```python
from build123d import *

# Parameters (mm, degrees)
SKETCH1_W           = 72.75
SKETCH1_H           = 35.5
BOSS_EXTRUDE1_DEPTH = 2
SKETCH7_W           = 10.759451316
SKETCH7_H           = 30
BOSS_EXTRUDE4_DEPTH = 4
SKETCH10_W          = 10.759451316
SKETCH10_H          = 10
BOSS_EXTRUDE5_DEPTH = 43.2
FILLET2_R           = 5
SKETCH12_W          = 72.75
SKETCH12_H          = 35.5
BOSS_EXTRUDE6_DEPTH = 2
FILLET4_R           = 2
SKETCH16_W          = 27.8
SKETCH16_H          = 6.7
BOSS_EXTRUDE8_DEPTH = 8
SKETCH19_R          = 1.45
CUT_EXTRUDE2_DEPTH  = 4
SKETCH20_R          = 0.45
CUT_EXTRUDE3_DEPTH  = 102.358708347
SKETCH21_R          = 3.1
CUT_EXTRUDE4_DEPTH  = 5


with BuildPart() as part:
    # Sketch1 → Boss-Extrude1 (new body)
    with BuildSketch(Plane(origin=(0, 0, 0), x_dir=(1, 0, 0), z_dir=(0, 1, 0))):
        with Locations((30.829669563, 14.626919984)):
            Rectangle(SKETCH1_W, SKETCH1_H)
    extrude(amount=BOSS_EXTRUDE1_DEPTH)

    # Sketch7 → Boss-Extrude4 (add)
    with BuildSketch(Plane(origin=(0, 2, 0), x_dir=(1, 0, 0), z_dir=(0, 1, 0))):
        with Locations((23.329669563, 47.376919984)):
            Rectangle(SKETCH7_W, SKETCH7_H)
    boss_extrude4 = extrude(amount=-BOSS_EXTRUDE4_DEPTH)

    # Mirror3: Boss-Extrude4 across plane
    add(boss_extrude4.mirror(Plane.XY.offset(-14.626919984)))

    # Sketch10 → Boss-Extrude5 (add)
    with BuildSketch(Plane(origin=(0, 2, 0), x_dir=(1, 0, 0), z_dir=(0, 1, 0))):
        with Locations((23.329669563, 57.376919984)):
            Rectangle(SKETCH10_W, SKETCH10_H)
    boss_extrude5 = extrude(amount=-BOSS_EXTRUDE5_DEPTH)

    # Mirror4: Boss-Extrude5 across plane
    add(boss_extrude5.mirror(Plane.XY.offset(-14.626919984)))

    # Fillet2
    fillet2_edges = [part.edges().sort_by_distance(p)[0] for p in [
        (23.329669563, 2, -62.376919984),
        (23.329669563, 2, 33.123080016),
    ]]
    fillet(fillet2_edges, radius=FILLET2_R)

    # Sketch12 → Boss-Extrude6 (add)
    with BuildSketch(Plane.XZ):
        with Locations((30.829669563, -14.626919984)):
            Rectangle(SKETCH12_W, SKETCH12_H)
    extrude(amount=BOSS_EXTRUDE6_DEPTH)

    # Fillet4
    fillet4_edges = [part.edges().sort_by_distance(p)[0] for p in [
        (67.204669563, 0, 3.123080016),
        (-5.545330437, 0, 3.123080016),
        (-5.545330437, 0, -32.376919984),
        (67.204669563, 0, -32.376919984),
    ]]
    fillet(fillet4_edges, radius=FILLET4_R)

    # Sketch16 → Boss-Extrude8 (add)
    with BuildSketch(Plane(origin=(67.204669563, 0, 0), x_dir=(0, 0, -1), z_dir=(1, 0, 0))):
        with Locations((14.626919984, 5.35)):
            Rectangle(SKETCH16_W, SKETCH16_H)
    extrude(amount=-BOSS_EXTRUDE8_DEPTH)

    # Sketch19 → Cut-Extrude2 (cut)
    with BuildSketch(Plane(origin=(67.204669563, 0, 0), x_dir=(0, 0, -1), z_dir=(1, 0, 0))):
        with Locations((17.826919984, 5.611929266)):
            Circle(SKETCH19_R)
        with Locations((11.426919984, 5.611929266)):
            Circle(SKETCH19_R)
    extrude(amount=-CUT_EXTRUDE2_DEPTH, mode=Mode.SUBTRACT)

    # Sketch20 → Cut-Extrude3 (cut, through all)
    with BuildSketch(Plane(origin=(0, 2, 0), x_dir=(1, 0, 0), z_dir=(0, 1, 0))):
        with Locations(Location((9.510831856, 26.461370287, 0), (0, 0, 270))):
            Circle(SKETCH20_R)
        with Locations(Location((12.050831856, 26.461370287, 0), (0, 0, 270))):
            Circle(SKETCH20_R)
        with Locations(Location((17.130831856, 26.461370287, 0), (0, 0, 270))):
            Circle(SKETCH20_R)
        with Locations(Location((47.485831856, 26.461370287, 0), (0, 0, 270))):
            Circle(SKETCH20_R)
        with Locations(Location((45.070831856, 26.461370287, 0), (0, 0, 270))):
            Circle(SKETCH20_R)
        with Locations(Location((37.450831856, 26.461370287, 0), (0, 0, 270))):
            Circle(SKETCH20_R)
        with Locations(Location((29.830831856, 26.461370287, 0), (0, 0, 270))):
            Circle(SKETCH20_R)
        with Locations(Location((14.590831856, 26.461370287, 0), (0, 0, 270))):
            Circle(SKETCH20_R)
        with Locations(Location((42.530831856, 26.461370287, 0), (0, 0, 270))):
            Circle(SKETCH20_R)
        with Locations(Location((39.990831856, 26.461370287, 0), (0, 0, 270))):
            Circle(SKETCH20_R)
        with Locations(Location((34.910831856, 26.461370287, 0), (0, 0, 270))):
            Circle(SKETCH20_R)
        with Locations(Location((32.370831856, 26.461370287, 0), (0, 0, 270))):
            Circle(SKETCH20_R)
        with Locations(Location((27.290831856, 26.461370287, 0), (0, 0, 270))):
            Circle(SKETCH20_R)
        with Locations(Location((24.750831856, 26.461370287, 0), (0, 0, 270))):
            Circle(SKETCH20_R)
        with Locations(Location((22.210831856, 26.461370287, 0), (0, 0, 270))):
            Circle(SKETCH20_R)
        with Locations(Location((19.670831856, 26.461370287, 0), (0, 0, 270))):
            Circle(SKETCH20_R)
        with Locations(Location((9.510831856, 2.561370287, 0), (0, 0, 90))):
            Circle(SKETCH20_R)
        with Locations(Location((12.050831856, 2.561370287, 0), (0, 0, 90))):
            Circle(SKETCH20_R)
        with Locations(Location((14.590831856, 2.561370287, 0), (0, 0, 90))):
            Circle(SKETCH20_R)
        with Locations(Location((17.130831856, 2.561370287, 0), (0, 0, 90))):
            Circle(SKETCH20_R)
        with Locations(Location((19.670831856, 2.561370287, 0), (0, 0, 90))):
            Circle(SKETCH20_R)
        with Locations(Location((22.210831856, 2.561370287, 0), (0, 0, 90))):
            Circle(SKETCH20_R)
        with Locations(Location((24.750831856, 2.561370287, 0), (0, 0, 90))):
            Circle(SKETCH20_R)
        with Locations(Location((29.830831856, 2.561370287, 0), (0, 0, 90))):
            Circle(SKETCH20_R)
        with Locations(Location((32.370831856, 2.561370287, 0), (0, 0, 90))):
            Circle(SKETCH20_R)
        with Locations(Location((34.910831856, 2.561370287, 0), (0, 0, 90))):
            Circle(SKETCH20_R)
        with Locations(Location((27.290831856, 2.561370287, 0), (0, 0, 90))):
            Circle(SKETCH20_R)
        with Locations(Location((39.990831856, 2.561370287, 0), (0, 0, 90))):
            Circle(SKETCH20_R)
        with Locations(Location((37.450831856, 2.561370287, 0), (0, 0, 90))):
            Circle(SKETCH20_R)
        with Locations(Location((42.530831856, 2.561370287, 0), (0, 0, 90))):
            Circle(SKETCH20_R)
        with Locations(Location((47.485831856, 2.561370287, 0), (0, 0, 90))):
            Circle(SKETCH20_R)
        with Locations(Location((45.070831856, 2.561370287, 0), (0, 0, 90))):
            Circle(SKETCH20_R)
    extrude(amount=-CUT_EXTRUDE3_DEPTH, mode=Mode.SUBTRACT)

    # Sketch21 → Cut-Extrude4 (cut)
    with BuildSketch(Plane.XZ.offset(41.2)):
        with Locations(Location((23.329669563, 28.123080016, 0), (0, 0, 270))):
            Circle(SKETCH21_R)
    cut_extrude4 = extrude(amount=-CUT_EXTRUDE4_DEPTH, mode=Mode.SUBTRACT)

    # Mirror5: Cut-Extrude4 across plane
    add(cut_extrude4.mirror(Plane.XY.offset(-14.626919984)), mode=Mode.SUBTRACT)


solid = part.part
```
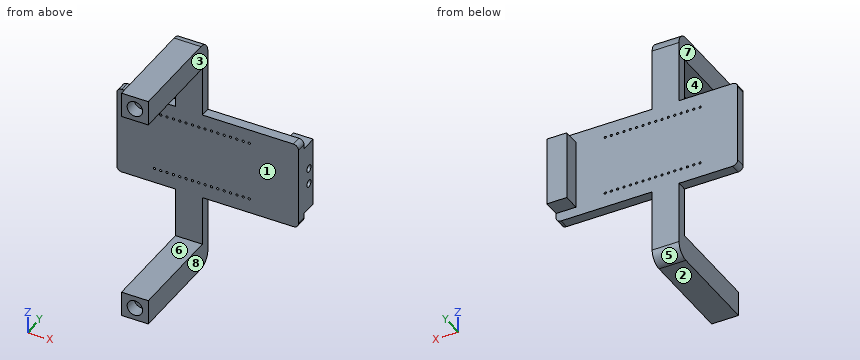
Verification items for the finished model (mm, model axes). Face numbers are marked on the shaded views. A direction names the side the tool comes from. Coordinates: 2 decimals unless noted, no trailing zeros. Write each loop counter-clockwise with the first axis right and the second up, starting at its lowest first coordinate (ties: lowest second). Pieces come first, ordered by that corner, then holes. Notation, with made-up numbers: M 17.5,50.25 L 21.5,50.25 A5 ccw 21.5,55.25 Z; hole C 9.5,56.5 d10. An arc over 180 degrees is marked long. Answer as a JSON object with one key per item and string values. Group by question number.
(1) Cross-section at D-D, the plane z = -40.5. Record the cut outline in (x, y).
(2) Release check for a two-part mould opening along Z. For the marked faces 1, 2, 3 and 4 record: +Z half, -Z half, draft (parallel to the pull), parting line (faces both ways), or undercut.
(3) Cross-section at B-B, the plane z = -21.5. Record the cut outline in (x, y), and give its area (3 significant figures).
(4) Tool access check on the marked faces 5, 6, 7 and 8. Record the directions out of +Z, -Z, +X, -X, +Y, -Y that give a thin tool (end or side, any length) a straight path to the whole face; none if there is none.
(5) Material ranges on line 1 (X direction, y = -29.5, z = 27); line 2 (X direction, y = 0.5, z = -30.5); line 3 (Y direction, x = 61, z = 0), recorded low to high.
(6) Cross-section at C-C, the plane x = -1. Record the cut outline in (y, z).
(7) Gauge pin test, flat ends, axial feed: pin 1 (2 mm diameter, centred on x = 6.5, y = -0.5, fed in from +Z); pin 2 (2 mm diameter, centred on x = 45, y = 0, fed in from -Z); pin 3 (15 mm diameter, centred on y = -28, z = -50.5, fed in from +X); pin 4 (4 mm diameter, centred on y = 5.61, z = -11.43, fed in from +X). Record the tip position at first contact, or that the pin passes through.
(8) Cross-section at A-A, the plane y = -22.5. Record the cut outline in (x, z), and give its area (3 significant figures).
Reply:
{
 "1": {"outline": "M 17.95,-2 L 28.71,-2 L 28.71,2 L 17.95,2 Z"},
 "2": {"face 1": "undercut", "face 2": "-Z half", "face 3": "draft", "face 4": "undercut"},
 "3": {"outline": "M -5.55,-2 L 67.2,-2 L 67.2,8.7 L 59.2,8.7 L 59.2,2 L -5.55,2 Z", "area": "345 mm²"},
 "4": {"face 5": "-Z, +X, -X, +Y", "face 6": "+X, -X, -Y", "face 7": "+Z, -X, +Y, -Y", "face 8": "-Z, +X, +Y, -Y"},
 "5": {"line 1": "17.95 to 28.71", "line 2": "-5.54 to 67.2", "line 3": "-2 to 2"},
 "6": {"outline": "M -2,-32.38 L 2,-32.38 L 2,3.12 L -2,3.12 Z"},
 "7": {"pin 1": "z = 3.12", "pin 2": "z = -32.38", "pin 3": "x = 28.71", "pin 4": "x = 67.2"},
 "8": {"outline": "M 17.95,-62.38 L 28.71,-62.38 L 28.71,-52.38 L 17.95,-52.38 Z; M 17.95,23.12 L 28.71,23.12 L 28.71,33.12 L 17.95,33.12 Z", "area": "215 mm²"}
}
